```python
from build123d import *

# Parameters (mm, degrees)
SKETCH_1_W          = 30
SKETCH_1_H          = 9
EXTRUDE_3_DEPTH     = 12
SKETCH_5_W          = 29
SKETCH_5_H          = 8
CUT_EXTRUDE_4_DEPTH = 11
EXTRUDE_5_DEPTH     = 1.25
FILLET_4_R          = 1


with BuildPart() as part:
    # 草图1 → 凸台-拉伸3 (new body)
    with BuildSketch(Plane(origin=(0, 0, 0), x_dir=(1, 0, 0), z_dir=(0, 1, 0))):
        with Locations((-0.5, -0.5)):
            Rectangle(SKETCH_1_W, SKETCH_1_H)
    extrude(amount=-EXTRUDE_3_DEPTH)

    # 草图5 → 切除-拉伸4 (cut)
    with BuildSketch(Plane(origin=(0, 0, 0), x_dir=(1, 0, 0), z_dir=(0, 1, 0))):
        Rectangle(SKETCH_5_W, SKETCH_5_H)
    extrude(amount=-CUT_EXTRUDE_4_DEPTH, mode=Mode.SUBTRACT)

    # 草图6 → 凸台-拉伸5 (add)
    with BuildSketch(Plane(origin=(0, 0, 0), x_dir=(1, 0, 0), z_dir=(0, 1, 0))):
        with BuildLine():
            Line((-17, 0), (-14, 0))
            ThreePointArc((-14, 0), (-13.707106781, -0.707106781), (-13, -1))
            Line((-13, -1), (-11, -1))
            ThreePointArc((-11, -1), (-10.292893219, -0.707106781), (-10, 0))
            Line((-10, 0), (-2.6, 0))
            ThreePointArc((-2.6, 0), (0, -2.6), (2.6, 0))
            Line((2.6, 0), (10, 0))
            ThreePointArc((10, 0), (10.292893219, -0.707106781), (11, -1))
            Line((11, -1), (13, -1))
            ThreePointArc((13, -1), (13.707106781, -0.707106781), (14, 0))
            Line((14, 0), (17, 0))
            Line((17, 0), (17, -5))
            ThreePointArc((17, -5), (16.560660172, -6.060660172), (15.5, -6.5))
            Line((15.5, -6.5), (-15.5, -6.5))
            ThreePointArc((-15.5, -6.5), (-16.560660172, -6.060660172), (-17, -5))
            Line((-17, -5), (-17, 0))
        make_face()
    extrude(amount=EXTRUDE_5_DEPTH)

    # 圆角4
    fillet_4_edges = [part.edges().sort_by_distance(p)[0] for p in [
        (-15.5, -12, 0.5),
        (-0.5, -12, 5),
        (-15.5, -6, 5),
    ]]
    fillet(fillet_4_edges, radius=FILLET_4_R)


solid = part.part
```
Source: CAD feature listing. Evaluate the final solid. Frame: model axes, mm. A direction names the side the tool comes from. Round coordinates to 2 decimals unless told otherwise and drop trailing zeros. Write each loop counter-clockwise with the first axis right and the second up, starting at its lowest first coordinate (ties: lowest second). Pieces come first, ordered by that corner, then holes. Notation, with made-up numbers: M 29,-2.75 L 85,-2.75 A27 cw 85,21.25 Z; hole C -11.75,78.5 d5. An arc over 180 degrees is marked long. Use CSV: the item, a comma, the result in double quotes. Start each with the question number.
Q1. Cut plane B-B on y = -3. Output: boundary loops of the cut face in (x, z).
Q2. Line query: line 1 (Y direction, x = -1.5, z = 3.5); line 2 (Z direction, x = -6, y = -4.5); line 3 (Y direction, x = 8.5, z = -1.25). Output: solid intervals per line, ascending. Write a range as from..to.
Q3. First-contact query: P1, Ø4, axis at y = -8.5, z = -1.5, coming from the -X side; P2, Ø1, axis at x = 12, y = -3, coming from the -Z side; P3, Ø2, axis at x = 9.5, z = -1.5, coming from the +Y side. Flat tips, straight axial feed; report the tip coordinate or a pass-through.
Q4. Cut plane C-C on x = 0. Output: boundary loops of the cut face in (y, z), plus the area to 3 significant figures.
Q5. Pull-direction query (X, two-part tool) for faces 5 (the face through (12, 1, 1)), 6 (the face through (-6, 1, 0)), 7 (the face through (-14.5, -5, 0)); classes: +X half, -X half, draft (parallel to the pull), parting line (faces both ways), or undercut.
Q6. Cut plane A-A on z = -2.75. Output: boundary loops of the cut face in (x, y).
Q7. Access query for faces 1 (the face through (0, -11, 0)), 2 (the face through (-16, 1, 0)), 3 (the face through (14.5, -7.7, 4.2)), 4 (the face through (10.285, 0.616, 0.699)). Directions: +Z, -Z, +X, -X, +Y, -Y. A direction counts if a zero-diameter tool reaches every point of the face in a straight line with its end or side. Return the directions, or none.
Q8. Cut plane D-D on z = 1.5. Output: boundary loops of the cut face in (x, y), plus the area to 3 significant figures.
Results found:
1,outline,"M -15.5,-4 L -14.5,-4 L -14.5,4 L 14.5,4 L 14.5,5 L -14.5,5 A1 ccw -15.5,4 Z"
2,line 1,"-12..-11, 0..1.25"
2,line 2,"4..5"
2,line 3,"-12..-11"
3,P1,"x = -15.5"
3,P2,"z = 4"
3,P3,"y = -11"
4,outline,"M -12,-4 L -11,-4 L -11,4 L 0,4 L 0,2.6 L 1.25,2.6 L 1.25,6.5 L 0,6.5 L 0,5 L -11,5 A1 ccw -12,4 Z"
4,area,"24.7 mm^2"
5,face 5,"undercut"
5,face 6,"draft"
5,face 7,"+X half"
6,outline,"M -15.5,-11 A1 ccw -14.5,-12 L 14.5,-12 L 14.5,-11 L -14.5,-11 L -14.5,0 L -15.5,0 Z"
7,face 1,"-Z, +X"
7,face 2,"-Z, +X, -X, +Y"
7,face 3,"+Z, -Z, +X, -Y"
7,face 4,"-Z, +Y"
8,outline,"M -17,0 L -15.5,0 L -15.5,-11 A1 ccw -14.5,-12 L 14.5,-12 L 14.5,-11 L -14.5,-11 L -14.5,0 L -2.12,0 L -2.12,1.25 L -17,1.25 Z; M 2.12,0 L 17,0 L 17,1.25 L 2.12,1.25 Z"
8,area,"78.0 mm^2"
